Input: part model. Units: mm. Frame: model coordinates. A direction names the side the tool comes from. Coordinates: 2 decimals unless noted, no trailing zeros. Write each loop counter-clockwise with the first axis right and the second up, starting at its lowest first coordinate (ties: lowest second). Pieces come first, ordered by that corner, then holes.
1) Section query A-A (x = 109.5). Output: boundary loops of the cut face in (y, z).
2) Set-up query: faces 1 (the cylindrical face through (85.02, -27.89, -27.76)), 2 (the flat face through (85, 25.22, -39)), 3 (the flat face through (85, -38, 25.22)). Return all of +Z, -Z, +X, -X, +Y, -Y with unobstructed straight access to the full face (end or side cutting, diameter ignored); none if empty.
3) Line query: L1, parallel to Y at x = 12, z = -34; L2, parallel to Z at x = 49, y = -0.5. Output: solid intervals per line, ascending.
4) Section query D-D (y = 16.5). Output: boundary loops of the cut face in (x, z) (3 decimals).
5) Draft query along Y for faces 4 (the cylindrical face through (85.02, 27.76, -27.89)), 5 (the cylindrical face through (7.888, 33.589, 38.076)), 6 (the flat face through (-4.375, 6, -6)). Return one class per face: pulls with the +Y half, pulls with the -Y half, needs draft (parallel to the pull), parting line crosses it, or undercut.
6) Section query C-C (z = 0). Output: boundary loops of the cut face in (x, y) (3 decimals).
7) Section query B-B (y = -32). Output: boundary loops of the cut face in (x, z).
8) Pin query (flat end, axial travel): pin 1 Ø4 at (y, z) = (-3, -2.5) entering from +X; pin 2 Ø9 at (y, z) = (-34.11, 34.11) entering from -X; pin 3 Ø7 at (x, y) = (106.5, -37.5) entering from -Z; pin 4 Ø5 at (y, z) = (34.11, -34.11) entering from -X. Return the tip coordinate at first contact, or that it passes through.
from build123d import *

# Parameters (mm, degrees)
F0_R     = 7
F1_DEPTH = 35
F0_R_2   = 30.10154
F2_DEPTH = 4.375
F3_DEPTH = 156
F0_R_3   = 4
F4_DEPTH = 16


with BuildPart() as f1:
    # F0 (on Right) → F1 (new body)
    with BuildSketch(Plane.YZ):
        Circle(F0_R)
    extrude(amount=-F1_DEPTH)

    # F0 (on Right) → F2 (join)
    with BuildSketch(Plane.YZ):
        Circle(F0_R_2)
        Circle(F0_R, mode=Mode.SUBTRACT)
    extrude(amount=-F2_DEPTH)

    # F0 (on Right) → F3 (join)
    with BuildSketch(Plane.YZ):
        with BuildLine():
            Line((-25.22, -43), (25.22, -43))
            Line((25.22, -43), (25.22, -34.11))
            ThreePointArc((25.22, -34.11), (27.8238207153, -27.8238207153), (34.11, -25.22))
            Line((34.11, -25.22), (43, -25.22))
            Line((43, -25.22), (43, 25.22))
            Line((43, 25.22), (34.11, 25.22))
            ThreePointArc((34.11, 25.22), (27.8238207153, 27.8238207153), (25.22, 34.11))
            Line((25.22, 34.11), (25.22, 43))
            Line((25.22, 43), (-25.22, 43))
            Line((-25.22, 43), (-25.22, 34.11))
            ThreePointArc((-25.22, 34.11), (-27.8238207153, 27.8238207153), (-34.11, 25.22))
            Line((-34.11, 25.22), (-43, 25.22))
            Line((-43, 25.22), (-43, -25.22))
            Line((-43, -25.22), (-34.11, -25.22))
            ThreePointArc((-34.11, -25.22), (-27.8238207153, -27.8238207153), (-25.22, -34.11))
            Line((-25.22, -34.11), (-25.22, -43))
        make_face()
        Circle(F0_R_2, mode=Mode.SUBTRACT)
        Circle(F0_R_2)
        Circle(F0_R, mode=Mode.SUBTRACT)
    extrude(amount=F3_DEPTH)

    # F0 (on Right) → F4 (join)
    with BuildSketch(Plane.YZ):
        with BuildLine():
            Line((-43, 34.11), (-43, 25.22))
            Line((-43, 25.22), (-34.11, 25.22))
            ThreePointArc((-34.11, 25.22), (-27.8238207153, 27.8238207153), (-25.22, 34.11))
            Line((-25.22, 34.11), (-25.22, 43))
            Line((-25.22, 43), (-34.11, 43))
            ThreePointArc((-34.11, 43), (-40.3961792847, 40.3961792847), (-43, 34.11))
        make_face()
        with Locations((-34.11, 34.11)):
            Circle(F0_R_3, mode=Mode.SUBTRACT)
        with BuildLine():
            Line((34.11, 25.22), (43, 25.22))
            Line((43, 25.22), (43, 34.11))
            ThreePointArc((43, 34.11), (40.3961792847, 40.3961792847), (34.11, 43))
            Line((34.11, 43), (25.22, 43))
            Line((25.22, 43), (25.22, 34.11))
            ThreePointArc((25.22, 34.11), (27.8238207153, 27.8238207153), (34.11, 25.22))
        make_face()
        with Locations((34.11, 34.11)):
            Circle(F0_R_3, mode=Mode.SUBTRACT)
        with BuildLine():
            Line((25.22, -43), (34.11, -43))
            ThreePointArc((34.11, -43), (40.3961792847, -40.3961792847), (43, -34.11))
            Line((43, -34.11), (43, -25.22))
            Line((43, -25.22), (34.11, -25.22))
            ThreePointArc((34.11, -25.22), (27.8238207153, -27.8238207153), (25.22, -34.11))
            Line((25.22, -34.11), (25.22, -43))
        make_face()
        with Locations((34.11, -34.11)):
            Circle(F0_R_3, mode=Mode.SUBTRACT)
        with BuildLine():
            Line((-34.11, -43), (-25.22, -43))
            Line((-25.22, -43), (-25.22, -34.11))
            ThreePointArc((-25.22, -34.11), (-27.8238207153, -27.8238207153), (-34.11, -25.22))
            Line((-34.11, -25.22), (-43, -25.22))
            Line((-43, -25.22), (-43, -34.11))
            ThreePointArc((-43, -34.11), (-40.3961792847, -40.3961792847), (-34.11, -43))
        make_face()
        with Locations((-34.11, -34.11)):
            Circle(F0_R_3, mode=Mode.SUBTRACT)
    extrude(amount=F4_DEPTH)


solid = f1.part
Answer:
1. outline: (-43, -25.22) - (-34.11, -25.22) arc R8.89 cw to (-25.22, -34.11) - (-25.22, -43) - (25.22, -43) - (25.22, -34.11) arc R8.89 cw to (34.11, -25.22) - (43, -25.22) - (43, 25.22) - (34.11, 25.22) arc R8.89 cw to (25.22, 34.11) - (25.22, 43) - (-25.22, 43) - (-25.22, 34.11) arc R8.89 cw to (-34.11, 25.22) - (-43, 25.22) - close; hole circle Ø14 at (0, 0)
2. face 1: -Z, +X, -Y
2. face 2: -Z, +X, +Y
2. face 3: +Z, +X, -Y
3. L1: y = -43 to -38.11, -30.11 to 30.11, 38.11 to 43
3. L2: z = -43 to -6.98, 6.98 to 43
4. outline: (-4.375, -25.176) - (0, -25.176) - (0, -43) - (156, -43) - (156, 43) - (0, 43) - (0, 25.176) - (-4.375, 25.176) - close
5. face 4: pulls with the +Y half
5. face 5: undercut
5. face 6: needs draft
6. outline: (-35, -7) - (-4.375, -7) - (-4.375, -30.102) - (0, -30.102) - (0, -43) - (156, -43) - (156, -7) - (0, -7) - (0, 7) - (156, 7) - (156, 43) - (0, 43) - (0, 30.102) - (-4.375, 30.102) - (-4.375, 7) - (-35, 7) - close
7. outline: (0, -43) - (16, -43) - (16, -37.51) - (0, -37.51) - close; (0, -30.71) - (16, -30.71) - (16, -25.47) - (156, -25.47) - (156, 25.47) - (16, 25.47) - (16, 30.71) - (0, 30.71) - close; (0, 37.51) - (16, 37.51) - (16, 43) - (0, 43) - close
8. pin 1: stops at x = 0
8. pin 2: stops at x = 0
8. pin 3: stops at z = -25.22
8. pin 4: passes through
